Source: CAD feature listing. Evaluate the final solid. Frame: model axes, mm. Face numbers are marked on the shaded views. A direction names the side the tool comes from. Give positions to 0.01 mm unless a question says otherwise; leave off trailing zeros. Write each loop counter-clockwise with the first axis right and the second up, starting at its lowest first coordinate (ties: lowest second). Pieces come first, ordered by that corner, then holes. Notation, with made-up numbers: (-23.5, 10) - (-3.5, 10) arc R19 cw to (-3.5, 17) - close; hole circle Ø7 at (-38, -35.5). An arc over 180 degrees is marked (long way). One line per question, with ' | ' between items. Start each with the question number.
(1) Access query for the marked faces 5, 6 and 7. Directions: +Z, -Z, +X, -X, +Y, -Y. A direction counts if a zero-diameter tool reaches every point of the face in a straight line with its end or side. Return the directions, or none.
(2) Section A-A, the plane y = 4. Return loops of the section in (x, z), plus the area to 3 significant figures.
(3) Pin query (flat end, axial travel): pin 1 (0.6 mm diameter, centred on y = 1, z = 1.5, fed in from -X); pin 2 (1.5 mm diameter, centred on x = 0.45, y = 4, fed in from +Z); pin 3 (1.6 mm diameter, centred on y = 1, z = 3.5, fed in from +X); pin 4 (3 mm diameter, centred on y = 7, z = 3.5, fed in from -X). Return the tip coordinate at first contact, or that it passes through.
(4) Section D-D, the plane y = 1. Return loops of the section in (x, z), plus the area to 3 significant figures.
(5) Ray query, line 1 (Y direction, x = 10.65, z = 1.25); line 2 (X direction, y = 3.75, z = 3.1); line 3 (X direction, y = 4.5, z = 2.3). Return the intervals inside material, ascending. Write a range as [from, to].
(6) Draft query along X for the marked faces 1, 2, 3 and 4. Return one class per face: +X half, -X half, draft (parallel to the pull), parting line (faces both ways), or undercut.
(7) Section C-C, the plane z = 2.8. Return loops of the section in (x, y).
(8) Section B-B, the plane x = 1. Return loops of the section in (y, z), plus the area to 3 significant figures.
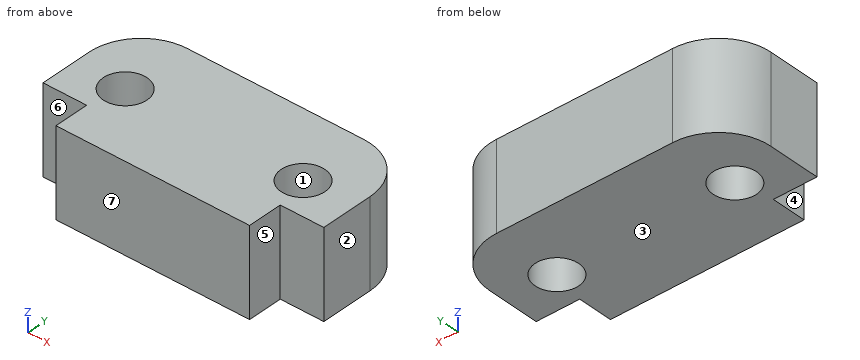
```python
from build123d import *

# Parameters (mm, degrees)
MODEL_R             = 1.25
BOSS_EXTRUDE1_DEPTH = 5


with BuildPart() as part:
    # Model → Boss-Extrude1 (new body)
    with BuildSketch(Plane.XY):
        with BuildLine():
            Line((0, 2), (-2.5, 2))
            Line((-2.5, 2), (-2.5, 4.995169548))
            ThreePointArc((-2.5, 4.995169548), (-1.621320344, 7.116489891), (0.5, 7.995169548))
            Line((0.5, 7.995169548), (10.6, 7.995169548))
            ThreePointArc((10.6, 7.995169548), (12.721320344, 7.116489891), (13.6, 4.995169548))
            Line((13.6, 4.995169548), (13.6, 2))
            Line((13.6, 2), (11.1, 2))
            Line((11.1, 2), (11.1, 0))
            Line((11.1, 0), (0, 0))
            Line((0, 0), (0, 2))
        make_face()
        with Locations((0.45, 4)):
            Circle(MODEL_R, mode=Mode.SUBTRACT)
        with Locations((10.65, 4)):
            Circle(MODEL_R, mode=Mode.SUBTRACT)
    extrude(amount=BOSS_EXTRUDE1_DEPTH)


solid = part.part
```
Check sheet entries:
1) face 5: +Z, -Z, +X, -Y | face 6: +Z, -Z, -X, -Y | face 7: +Z, -Z, +X, -X, -Y
2) outline: (-2.5, 0) - (-0.8, 0) - (-0.8, 5) - (-2.5, 5) - close; (1.7, 0) - (9.4, 0) - (9.4, 5) - (1.7, 5) - close; (11.9, 0) - (13.6, 0) - (13.6, 5) - (11.9, 5) - close | area: 55.5 mm²
3) pin 1: x = 0 | pin 2: through | pin 3: x = 11.1 | pin 4: x = -2.46
4) outline: (0, 0) - (11.1, 0) - (11.1, 5) - (0, 5) - close | area: 55.5 mm²
5) line 1: [0, 2.75], [5.25, 7.99] | line 2: [-2.5, -0.77], [1.67, 9.43], [11.87, 13.6] | line 3: [-2.5, -0.7], [1.6, 9.5], [11.8, 13.6]
6) face 1: undercut | face 2: +X half | face 3: draft | face 4: -X half
7) outline: (-2.5, 2) - (0, 2) - (0, 0) - (11.1, 0) - (11.1, 2) - (13.6, 2) - (13.6, 5) arc R3 ccw to (10.6, 8) - (0.5, 8) arc R3 ccw to (-2.5, 5) - close; hole circle Ø2.5 at (0.45, 4); hole circle Ø2.5 at (10.65, 4)
8) outline: (0, 0) - (2.88, 0) - (2.88, 5) - (0, 5) - close; (5.12, 0) - (8, 0) - (8, 5) - (5.12, 5) - close | area: 28.8 mm²
